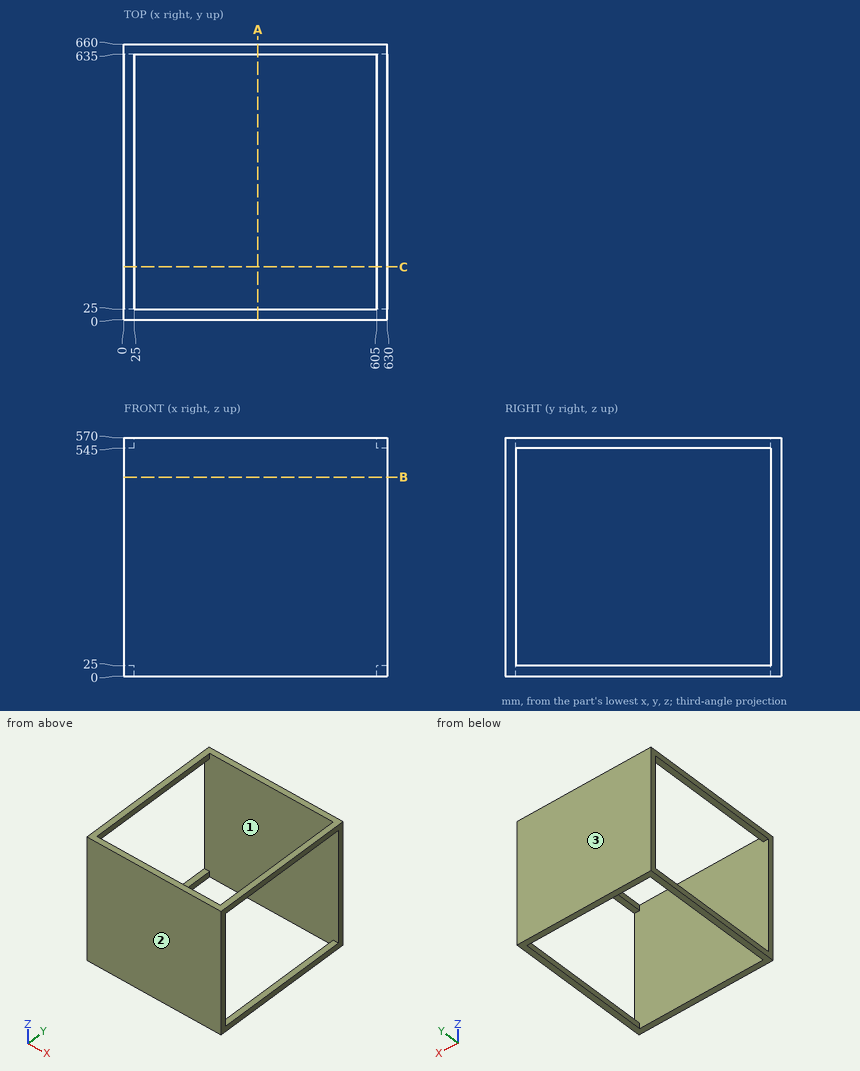
Study the drawing (mm; zero at the part's minimum x, y, z) and answer. Round coordinates to 2 decimals unless told otherwise and drop trailing zeros. Write each loop counter-clockwise with the first axis right and the second up, starting at its lowest first coordinate (ties: lowest second). Pieces come first, ordered by that corner, then holes. Notation, with made-up numbers: (-40, 66.5) -> (10, 66.5) arc R14 ccw to (10, 85.5) -> close; hole circle Ø9 at (42.5, 58). An arc over 180 degrees is marked (long way). Use CSV: the item, a comma, the result in double quotes. Start each with the question number.
(1) Section C-C on y = 126.5 is taken. Give the vertices of the cut face in (x, z).
(2) Section B-B on z = 476 is taken. Give the vertices of the cut face in (x, y), then the cut area to 3 significant figures.
(3) The mould has two halves that part along Y. Classify the marked faces 1, 2 and 3: released by +Y, released by -Y, zero draft, split by the parting line, or undercut.
(4) Consider L1, parallel to Y at x = 281, z = 356. Determine where the line is inside the solid, lowest interval first. Write a range as from..to.
(5) Section A-A on x = 320.5 is taken. Give the vertices of the cut face in (y, z).
A:
1,outline,"(0, 0) -> (25, 0) -> (25, 25) -> (0, 25) -> close; (0, 545) -> (25, 545) -> (25, 570) -> (0, 570) -> close; (605, 0) -> (630, 0) -> (630, 25) -> (605, 25) -> close; (605, 545) -> (630, 545) -> (630, 570) -> (605, 570) -> close"
2,outline,"(0, 0) -> (630, 0) -> (630, 25) -> (0, 25) -> close; (0, 635) -> (630, 635) -> (630, 660) -> (0, 660) -> close"
2,area,"31,500 mm²"
3,face 1,"undercut"
3,face 2,"released by -Y"
3,face 3,"released by +Y"
4,L1,"y = 0..25, 635..660"
5,outline,"(0, 0) -> (25, 0) -> (25, 570) -> (0, 570) -> close; (635, 0) -> (660, 0) -> (660, 570) -> (635, 570) -> close"
